```python
from build123d import *

# Parameters (mm, degrees)
F0_R      = 1.75
F1_DEPTH  = 4
F2_DEPTH  = 14
F1_FACE_W = 31
F1_FACE_H = 4
F3_DEPTH  = 28
F4_W      = 31
F4_H      = 4
F5_DEPTH  = 24
F7_W      = 31
F7_H      = 4
F8_DEPTH  = 24
F6_W      = 31
F6_H      = 4
F9_DEPTH  = 20


with BuildPart() as f1:
    # F0 (on Top) → F1 (new body)
    with BuildSketch(Plane.XY):
        with BuildLine():
            ThreePointArc((-4.149364, -27.437859), (-0.61383, -25.973393), (0.850636, -22.437859))
            ThreePointArc((0.850636, -22.437859), (-0.61383, -18.902325), (-4.149364, -17.437859))
            ThreePointArc((-4.149364, -17.437859), (-9.149364, -22.437859), (-4.149364, -27.437859))
        make_face()
        with Locations((-4.149364, -22.437859)):
            Circle(F0_R, mode=Mode.SUBTRACT)
        with BuildLine():
            ThreePointArc((-4.149364, -17.437859), (-0.61383, -18.902325), (0.850636, -22.437859))
            Line((0.850636, -22.437859), (21.850636, -22.437859))
            ThreePointArc((21.850636, -22.437859), (23.315102, -18.902325), (26.850636, -17.437859))
            Line((26.850636, -17.437859), (-4.149364, -17.437859))
        make_face()
        with BuildLine():
            ThreePointArc((26.850636, -17.437859), (23.315102, -18.902325), (21.850636, -22.437859))
            ThreePointArc((21.850636, -22.437859), (23.315102, -25.973393), (26.850636, -27.437859))
            ThreePointArc((26.850636, -27.437859), (30.38617, -25.973393), (31.850636, -22.437859))
            ThreePointArc((31.850636, -22.437859), (30.38617, -18.902325), (26.850636, -17.437859))
        make_face()
        with BuildLine():
            ThreePointArc((28.600636, -22.437859), (26.850636, -24.187859), (25.100636, -22.437859))
            ThreePointArc((25.100636, -22.437859), (26.850636, -20.687859), (28.600636, -22.437859))
        make_face(mode=Mode.SUBTRACT)
        with BuildLine():
            Line((21.850636, -22.437859), (0.850636, -22.437859))
            ThreePointArc((0.850636, -22.437859), (-0.61383, -25.973393), (-4.149364, -27.437859))
            Line((-4.149364, -27.437859), (26.850636, -27.437859))
            ThreePointArc((26.850636, -27.437859), (23.315102, -25.973393), (21.850636, -22.437859))
        make_face()
    extrude(amount=F1_DEPTH)

    # F0 (on Top) → F2 (join)
    with BuildSketch(Plane.XY):
        with BuildLine():
            ThreePointArc((-4.149364, -27.437859), (-0.61383, -25.973393), (0.850636, -22.437859))
            ThreePointArc((0.850636, -22.437859), (-0.61383, -18.902325), (-4.149364, -17.437859))
            ThreePointArc((-4.149364, -17.437859), (-9.149364, -22.437859), (-4.149364, -27.437859))
        make_face()
        with Locations((-4.149364, -22.437859)):
            Circle(F0_R, mode=Mode.SUBTRACT)
        with BuildLine():
            ThreePointArc((26.850636, -17.437859), (23.315102, -18.902325), (21.850636, -22.437859))
            ThreePointArc((21.850636, -22.437859), (23.315102, -25.973393), (26.850636, -27.437859))
            ThreePointArc((26.850636, -27.437859), (30.38617, -25.973393), (31.850636, -22.437859))
            ThreePointArc((31.850636, -22.437859), (30.38617, -18.902325), (26.850636, -17.437859))
        make_face()
        with BuildLine():
            ThreePointArc((28.600636, -22.437859), (26.850636, -24.187859), (25.100636, -22.437859))
            ThreePointArc((25.100636, -22.437859), (26.850636, -20.687859), (28.600636, -22.437859))
        make_face(mode=Mode.SUBTRACT)
    extrude(amount=F2_DEPTH)

    # F1_face (on face) → F3 (join)
    with BuildSketch(Plane(origin=(11.350636, -27.437859, 2), x_dir=(1, 0, 0), z_dir=(0, -1, 0))):
        Rectangle(F1_FACE_W, F1_FACE_H)
    extrude(amount=F3_DEPTH)

    # F4 (on face) → F5 (join)
    with BuildSketch(Plane(origin=(0, 0, 0), x_dir=(1, 0, 0), z_dir=(0, 0, -1))):
        with Locations((11.350636, 53.437859)):
            Rectangle(F4_W, F4_H)
    extrude(amount=F5_DEPTH)

    # F7 (on face) → F8 (join)
    with BuildSketch(Plane(origin=(0, 0, 0), x_dir=(1, 0, 0), z_dir=(0, 0, -1))):
        with Locations((11.350636, 29.437859)):
            Rectangle(F7_W, F7_H)
    extrude(amount=F8_DEPTH)

    # F6 (on face) → F9 (join, through all)
    with BuildSketch(Plane(origin=(0, -51.437859, 0), x_dir=(-1, 0, 0), z_dir=(0, 1, 0))):
        with Locations((-11.350636, -22)):
            Rectangle(F6_W, F6_H)
    extrude(amount=F9_DEPTH)


solid = f1.part
```
Read the model definition and answer for the solid it produces. Units are mm, in the model's axes. A direction names the side the tool comes from. Coordinates: 2 decimals unless noted, no trailing zeros. Loops run counter-clockwise (first coordinate to the right, second up) from the corner with the lowest first, then second, coordinate; pieces in that order, holes last. Notation, with made-up numbers: (52.25, 64.25) - (85.25, 64.25) arc R31 cw to (85.25, 94.25) - close; hole circle Ø4 at (36, 37). An arc over 180 degrees is marked (long way). Answer in a Markdown table with one row per item.
1. Straight lines are drawn through the part: line 1 (Y direction, x = 7, z = -5); line 2 (Z direction, x = -2.5, y = -33); line 3 (Z direction, x = 11, y = -25). For each, find the intervals that lie inside material, in ascending order.
Conclusion:
| item | result |
|---|---|
| line 1 | y = -55.44 to -51.44, -31.44 to -27.44 |
| line 2 | z = -24 to -20, 0 to 4 |
| line 3 | z = 0 to 4 |
2. Given pin 1 (14 mm diameter, centred on y = -35.5, z = -5, fed in from -X); pin 2 (11 mm diameter, centred on x = 21.5, y = -20.5, fed in from -Z); pin 3 (3 mm diameter, centred on y = -27.5, z = 7.5, fed in from +X); pin 4 (8.5 mm diameter, centred on y = -37.5, z = -9.5, fed in from +X), each flat-ended and moving along its own axis, determine where each tip first touches the part or whether it passes through.
Conclusion:
| item | result |
|---|---|
| pin 1 | stops at x = -4.15 |
| pin 2 | stops at z = 0 |
| pin 3 | stops at x = 30.36 |
| pin 4 | passes through |
3. Find section C-C, the plane y = -44. Write down the section's boundary in (x, z), then the cut area to 3 significant figures.
Conclusion:
| item | result |
|---|---|
| outline | (-4.15, -24) - (26.85, -24) - (26.85, -20) - (-4.15, -20) - close; (-4.15, 0) - (26.85, 0) - (26.85, 4) - (-4.15, 4) - close |
| area | 248 mm² |
4. Find section B-B, the plane z = -3.5. Write down the section's boundary in (x, y), then the cut area to 3 significant figures.
Conclusion:
| item | result |
|---|---|
| outline | (-4.15, -55.44) - (26.85, -55.44) - (26.85, -51.44) - (-4.15, -51.44) - close; (-4.15, -31.44) - (26.85, -31.44) - (26.85, -27.44) - (-4.15, -27.44) - close |
| area | 248 mm² |
5. Find section A-A, the plane z = 11.5. Write down the section's boundary in (x, y), then the cut area to 3 significant figures.
Conclusion:
| item | result |
|---|---|
| outline | circle Ø10 at (-4.15, -22.44); circle Ø10 at (26.85, -22.44); hole circle Ø3.5 at (-4.15, -22.44); hole circle Ø3.5 at (26.85, -22.44) |
| area | 138 mm² |
6. Find section D-D, the plane x = 6.5. Write down the section's boundary in (y, z).
Conclusion:
| item | result |
|---|---|
| outline | (-55.44, -24) - (-27.44, -24) - (-27.44, 0) - (-17.44, 0) - (-17.44, 4) - (-55.44, 4) - close; hole (-51.44, -20) - (-31.44, -20) - (-31.44, 0) - (-51.44, 0) - close |
7. Which of the six approach directions +Z, -Z, +X, -X, +Y, -Y give full straight-line access (tool end or side, diameter ignored) to faces 5 (the face through (11, -22, 0)), 6 (the face through (12, -17.438, 2)), 7 (the face through (12, -42, -24)), 8 (the face through (-4.149, -42, -23)), 9 (the face through (11, -41, 0))?
Conclusion:
| item | result |
|---|---|
| face 5 | -Z, +X, -X, +Y |
| face 6 | +Z, -Z, +X, -X, +Y |
| face 7 | -Z, +X, -X, +Y, -Y |
| face 8 | +Z, -Z, -X, -Y |
| face 9 | +X, -X |
8. Determine the mould class of faces 1 (the face through (11, -31.438, -10)), 2 (the face through (11, -55.438, -10)), 3 (the face through (26.851, -42, -23)), 4 (the face through (11, -27.438, -12)) for opening direction Y: +Y half, -Y half, draft (parallel to the pull), parting line (faces both ways), or undercut.
Conclusion:
| item | result |
|---|---|
| face 1 | undercut |
| face 2 | -Y half |
| face 3 | draft |
| face 4 | +Y half |
